Can you work these out from the model? Positions are in its coordinate system, mm. A direction names the side the tool comes from. Round coordinates to 2 decimals unless told otherwise and drop trailing zeros. Loops run counter-clockwise (first coordinate to the right, second up) from the corner with the lowest first, then second, coordinate; pieces in that order, holes last. Notation, with made-up numbers: (-4.75, -17) -> (51.25, -17) arc R5 cw to (51.25, -11) -> close; hole circle Ø11 at (80, 53.25). An arc over 180 degrees is marked (long way). Write item = value, one per line.
from build123d import *

# Parameters (mm, degrees)
SKETCH1_R           = 39.751
BOSS_EXTRUDE1_DEPTH = 103.124
SKETCH2_R           = 17.4625
BOSS_EXTRUDE2_DEPTH = 2.54
SKETCH3_R           = 6.35
BOSS_EXTRUDE3_DEPTH = 44.45
SKETCH4_R           = 2.159
CUT_EXTRUDE1_DEPTH  = 44.45


with BuildPart() as part:
    # Sketch1 → Boss-Extrude1 (new body)
    with BuildSketch(Plane(origin=(0, 0, 0), x_dir=(1, 0, 0), z_dir=(0, 1, 0))):
        Circle(SKETCH1_R)
    extrude(amount=BOSS_EXTRUDE1_DEPTH)

    # Sketch2 → Boss-Extrude2 (add)
    with BuildSketch(Plane(origin=(0, 103.124, 0), x_dir=(1, 0, 0), z_dir=(0, 1, 0))):
        Circle(SKETCH2_R)
    extrude(amount=BOSS_EXTRUDE2_DEPTH)

    # Sketch3 → Boss-Extrude3 (add)
    with BuildSketch(Plane(origin=(0, 105.664, 0), x_dir=(1, 0, 0), z_dir=(0, 1, 0))):
        Circle(SKETCH3_R)
    extrude(amount=BOSS_EXTRUDE3_DEPTH)

    # Sketch4 → Cut-Extrude1 (cut)
    with BuildSketch(Plane(origin=(0, 103.124, 0), x_dir=(1, 0, 0), z_dir=(0, 1, 0))):
        with Locations((0, 25)):
            Circle(SKETCH4_R)
        with Locations((25, 0)):
            Circle(SKETCH4_R)
        with Locations((0, -25)):
            Circle(SKETCH4_R)
        with Locations((-25, 0)):
            Circle(SKETCH4_R)
    extrude(amount=-CUT_EXTRUDE1_DEPTH, mode=Mode.SUBTRACT)


solid = part.part
1. I need wall thicknesses on line 1 (X direction, y = 84, z = 0); line 2 (Z direction, x = -0.5, y = 91). Which ranges of each line are inside material? Lowest first, please. Write a range as [from, to].
Entries:
line_1 = [-39.75, -27.16], [-22.84, 22.84], [27.16, 39.75]
line_2 = [-39.75, -27.1], [-22.9, 22.9], [27.1, 39.75]
2. Suppose I cut it at B-B, the plane x = 0. List the corners of the cut face in (y, z) for me, and give its area (3 significant figures).
Entries:
outline = (0, -39.75) -> (103.12, -39.75) -> (103.12, -27.16) -> (58.67, -27.16) -> (58.67, -22.84) -> (103.12, -22.84) -> (103.12, -17.46) -> (105.66, -17.46) -> (105.66, -6.35) -> (150.11, -6.35) -> (150.11, 6.35) -> (105.66, 6.35) -> (105.66, 17.46) -> (103.12, 17.46) -> (103.12, 22.84) -> (58.67, 22.84) -> (58.67, 27.16) -> (103.12, 27.16) -> (103.12, 39.75) -> (0, 39.75) -> close
area = 8,470 mm²
3. We'd pull the mould along Z, two halves only. Please class faces 3 (the flat face through (0, 58.674, 25)), 4 (the cylindrical face through (-13.858, 104.376, 10.626)), 5 (the flat face through (0, 150.114, 0)): released by +Z, released by -Z, zero draft, split by the parting line, or undercut.
Entries:
face_3 = undercut
face_4 = split by the parting line
face_5 = zero draft
4. Suppose I cut it at C-C, the plane y = 46.5. List the corners of the cut face in (x, z) for me.
Entries:
outline = circle Ø79.5 at (0, 0)
5. I'm going to push flat-ended pins straight in: pin 1 (3.5 mm diameter, centred on x = -1, z = 25, fed in from +Y); pin 2 (12 mm diameter, centred on y = 33.5, z = 19, fed in from -X); pin 3 (4 mm diameter, centred on x = 0, z = -25, fed in from +Y). Where does each tip first touch, or does it pass through?
Entries:
pin_1 = 103.12
pin_2 = -37.57
pin_3 = 58.67
6. Suppose I cut it at D-D, the plane x = -25. List the corners of the cut face in (y, z) for me, and give its area (3 significant figures).
Entries:
outline = (0, -30.91) -> (103.12, -30.91) -> (103.12, -2.16) -> (58.67, -2.16) -> (58.67, 2.16) -> (103.12, 2.16) -> (103.12, 30.91) -> (0, 30.91) -> close
area = 6,180 mm²
7. Suppose I cut it at A-A, the plane z = 0. List the corners of the cut face in (x, y) for me, and give its area (3 significant figures).
Entries:
outline = (-39.75, 0) -> (39.75, 0) -> (39.75, 103.12) -> (27.16, 103.12) -> (27.16, 58.67) -> (22.84, 58.67) -> (22.84, 103.12) -> (17.46, 103.12) -> (17.46, 105.66) -> (6.35, 105.66) -> (6.35, 150.11) -> (-6.35, 150.11) -> (-6.35, 105.66) -> (-17.46, 105.66) -> (-17.46, 103.12) -> (-22.84, 103.12) -> (-22.84, 58.67) -> (-27.16, 58.67) -> (-27.16, 103.12) -> (-39.75, 103.12) -> close
area = 8,470 mm²
8. For faces 1 (the flat face through (0, 58.674, -25)), 2 (the flat face through (-1, 0, -1)), which set-ups out of +Z, -Z, +X, -X, +Y, -Y let a thin tool reach every point of the face, with its end or its side?
Entries:
face_1 = +Y
face_2 = +Z, -Z, +X, -X, -Y
